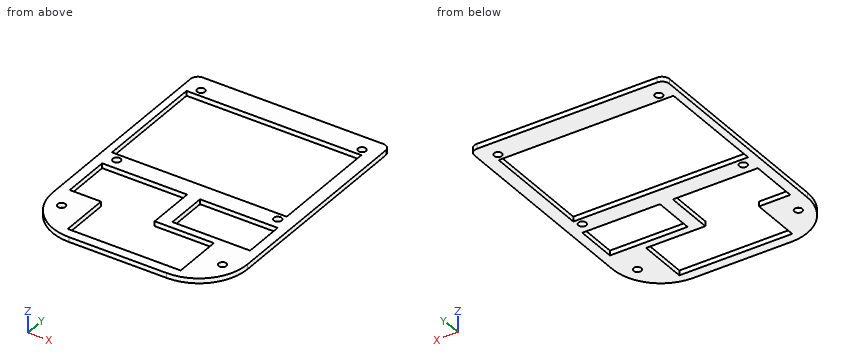
from build123d import *

# Parameters (mm, degrees)
SKETCH1_W                      = 80.3
SKETCH1_H                      = 66
BOSS_EXTRUDE1_DEPTH            = 2
F_3_2_3_2_DIAMETER_HOLE1_D     = 3.2
FILLET1_R                      = 3
SKETCH4_W                      = 80.3
SKETCH4_H                      = 2
BOSS_EXTRUDE2_DEPTH            = 42
FILLET2_R                      = 20
F_3_2_3_2_DIAMETER_HOLE2_D     = 3.2
F_3_2_3_2_DIAMETER_HOLE2_DEPTH = 60
F_3_2_3_2_DIAMETER_HOLE2_TIP   = 0.96137699
SKETCH7_W                      = 72
SKETCH7_H                      = 46
CUT_EXTRUDE1_DEPTH             = 3
SKETCH10_W                     = 35
SKETCH10_H                     = 20
SKETCH10_W_2                   = 32
SKETCH10_H_2                   = 17
CUT_EXTRUDE3_DEPTH             = 3


with BuildPart() as part:
    # Sketch1 → Boss-Extrude1 (new body)
    with BuildSketch(Plane.XY):
        with Locations((40.15, 33)):
            Rectangle(SKETCH1_W, SKETCH1_H)
    extrude(amount=BOSS_EXTRUDE1_DEPTH)

    # Ø3.2 (3.2) Diameter Hole1 (through all)
    with Locations(Plane.XY.offset(2)):
        with Locations((7, 59), (73.3, 59), (73.3, 7), (7, 7)):
            Hole(F_3_2_3_2_DIAMETER_HOLE1_D / 2)

    # Fillet1
    fillet1_edges = [part.edges().sort_by_distance(p)[0] for p in [
        (0, 66, 1),
        (80.3, 66, 1),
    ]]
    fillet(fillet1_edges, radius=FILLET1_R)

    # Sketch4 → Boss-Extrude2 (add)
    with BuildSketch(Plane.XZ):
        with Locations((40.15, 1)):
            Rectangle(SKETCH4_W, SKETCH4_H)
    extrude(amount=BOSS_EXTRUDE2_DEPTH)

    # Fillet2
    fillet2_edges = [part.edges().sort_by_distance(p)[0] for p in [
        (0, -42, 1),
        (80.3, -42, 1),
    ]]
    fillet(fillet2_edges, radius=FILLET2_R)

    # Ø3.2 (3.2) Diameter Hole2
    with Locations(Plane.XY.offset(2)):
        with Locations((7, -27), (73.3, -27)):
            Hole(F_3_2_3_2_DIAMETER_HOLE2_D / 2, depth=F_3_2_3_2_DIAMETER_HOLE2_DEPTH)
            with Locations((0, 0, -(F_3_2_3_2_DIAMETER_HOLE2_DEPTH + F_3_2_3_2_DIAMETER_HOLE2_TIP / 2))):  # 118° drill point
                Cone(0, F_3_2_3_2_DIAMETER_HOLE2_D / 2, F_3_2_3_2_DIAMETER_HOLE2_TIP, mode=Mode.SUBTRACT)

    # Sketch7 → Cut-Extrude1 (cut, through all)
    with BuildSketch(Plane.XY.offset(2)):
        with Locations((39, 33)):
            Rectangle(SKETCH7_W, SKETCH7_H)
    extrude(amount=-CUT_EXTRUDE1_DEPTH, mode=Mode.SUBTRACT)

    # Sketch10 → Cut-Extrude3 (cut, through all)
    with BuildSketch(Plane.XY.offset(2)):
        with Locations((21.5, -7.5)):
            Rectangle(SKETCH10_W, SKETCH10_H)
        Polygon((63.4, -17.5), (39, -17.5), (16.9, -17.5), (16.9, -38), (63.4, -38), align=None)
        with Locations((60.3, -6)):
            Rectangle(SKETCH10_W_2, SKETCH10_H_2)
    extrude(amount=-CUT_EXTRUDE3_DEPTH, mode=Mode.SUBTRACT)


solid = part.part
For this review, take the finished solid that the model builds, in its own axes (mm). Coordinates: 2 decimals unless noted, no trailing zeros. Order: outer loops, then holes, each group sorted by start corner. A loop starts at its lowest first (then second) coordinate and runs counter-clockwise, first axis right, second up. Notation, with made-up numbers: (-3.5, 50.5) -> (50.5, 50.5) arc R9 cw to (50.5, 61.5) -> close; hole circle Ø10 at (66, -16). An arc over 180 degrees is marked (long way). Return JSON: item names as keys, results as strings.
1. We need section D-D on y = 59. Write out the cut boundary in (x, z).
Answer block:
{"outline": "(0, 0) -> (5.4, 0) -> (5.4, 2) -> (0, 2) -> close; (8.6, 0) -> (71.7, 0) -> (71.7, 2) -> (8.6, 2) -> close; (74.9, 0) -> (80.3, 0) -> (80.3, 2) -> (74.9, 2) -> close"}
2. We need section A-A on y = 40. Write out the cut boundary in (x, z).
Answer block:
{"outline": "(0, 0) -> (3, 0) -> (3, 2) -> (0, 2) -> close; (75, 0) -> (80.3, 0) -> (80.3, 2) -> (75, 2) -> close"}
3. For line 1 (Y direction, x = 45, z = 0.3); line 2 (Y direction, x = 24, z = 1.65); line 3 (X direction, y = 1, z = 0.25), list the stretches that pass through material, from the lowest coordinate up. Write a range as from..to.
Answer block:
{"line 1": "-42..-38, -17.5..-14.5, 2.5..10, 56..66", "line 2": "-42..-38, 2.5..10, 56..66", "line 3": "0..4, 39..44.3, 76.3..80.3"}
4. For pin 1 Ø12 at (x, y) = (59, 49) entering from -Z (3 decimals), flat-tipped, find the tip position at first contact; note if it passes through.
Answer block:
{"pin 1": "through"}
5. We need section B-B on z = 1.7. State how many separate pieces and enclosed holes the cut face has, and give its area (3 significant figures).
Answer block:
{"separate pieces": "1", "enclosed holes": "9", "area": "2,940 mm²"}
6. We need section C-C on x = 26.5. Write out the cut boundary in (y, z).
Answer block:
{"outline": "(-42, 0) -> (-38, 0) -> (-38, 2) -> (-42, 2) -> close; (2.5, 0) -> (10, 0) -> (10, 2) -> (2.5, 2) -> close; (56, 0) -> (66, 0) -> (66, 2) -> (56, 2) -> close"}
